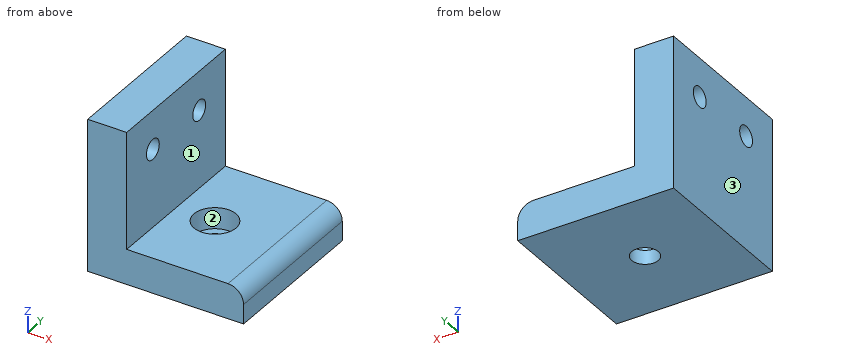
```python
from build123d import *

# Parameters (mm, degrees)
SKETCH_W        = 20
SKETCH_H        = 20
PAD_DEPTH       = 4.5
SKETCH001_R     = 1.7
POCKET_DEPTH    = 5
SKETCH002_R     = 2.7
POCKET001_DEPTH = 2.7
SKETCH003_W     = 5
SKETCH003_H     = 20
PAD001_DEPTH    = 15
SKETCH004_R     = 1.3
POCKET002_DEPTH = 5
FILLET_R        = 2


with BuildPart() as part:
    # Sketch → Pad (new body)
    with BuildSketch(Plane.XY):
        Rectangle(SKETCH_W, SKETCH_H)
    extrude(amount=PAD_DEPTH)

    # Sketch001 (on Face6 of Pad) → Pocket (cut)
    with BuildSketch(Plane.XY.offset(4.5)):
        Circle(SKETCH001_R)
    extrude(amount=-POCKET_DEPTH, mode=Mode.SUBTRACT)

    # Sketch002 (on Face5 of Pocket) → Pocket001 (cut)
    with BuildSketch(Plane.XY.offset(4.5)):
        Circle(SKETCH002_R)
    extrude(amount=-POCKET001_DEPTH, mode=Mode.SUBTRACT)

    # Sketch003 (on Face5 of Pocket001) → Pad001 (join)
    with BuildSketch(Plane.XY.offset(4.5)):
        with Locations((-7.5, 0)):
            Rectangle(SKETCH003_W, SKETCH003_H)
    extrude(amount=PAD001_DEPTH)

    # Sketch004 (on Face10 of Pad001) → Pocket002 (cut)
    with BuildSketch(Plane.YZ.offset(-5)):
        with Locations((-4.7, 14.5)):
            Circle(SKETCH004_R)
        with Locations((4.7, 14.5)):
            Circle(SKETCH004_R)
    extrude(amount=-POCKET002_DEPTH, mode=Mode.SUBTRACT)

    # Fillet
    fillet_edges = [part.edges().sort_by_distance(p)[0] for p in [
        (10, 0, 4.5),
    ]]
    fillet(fillet_edges, radius=FILLET_R)


solid = part.part
```
Here's how the part is built. I have some questions about the finished solid (model axes, mm). Face numbers are marked on the shaded views. A direction names the side the tool comes from. Coordinates: 2 decimals unless noted, no trailing zeros. Order: outer loops, then holes, each group sorted by start corner. A loop starts at its lowest first (then second) coordinate and runs counter-clockwise, first axis right, second up.
1) Will these pins go through, and if not, where does the flat tip stop? pin 1 (8 mm diameter, centred on x = 3, y = -6.5, fed in from +Z); pin 2 (7.5 mm diameter, centred on y = 2.5, z = 13, fed in from +X).
2) I need wall thicknesses on line 1 (Y direction, x = 0, z = 1.15); line 2 (Y direction, x = 0, z = 3); line 3 (Z direction, x = -8, y = 4.7). Which ranges of each line are inside material? Lowest first, please.
3) Imagine slicing it at C-C on z = 14.5. List the corners of the cut face in (x, y) for me.
4) Imagine slicing it at B-B on x = 0. List the corners of the cut face in (y, z) for me, and give its area (3 significant figures).
5) Which directions (+Z, -Z, +X, -X, +Y, -Y) give clear straight access to the entire face, cutting with the end or side of a thin tool? Please do the marked faces 1, 2 and 3.
6) Imagine slicing it at D-D on x = -6.75. List the corners of the cut face in (y, z) for me, and give its area (3 significant figures).
7) Imagine slicing it at A-A on y = -4.7. List the corners of the cut face in (x, z) for me, and give its area (3 significant figures).
Response values:
1. pin 1: stops at z = 4.5
1. pin 2: stops at x = -5
2. line 1: y = -10 to -1.7, 1.7 to 10
2. line 2: y = -10 to -2.7, 2.7 to 10
2. line 3: z = 0 to 13.2, 15.8 to 19.5
3. outline: (-10, -10) - (-5, -10) - (-5, -6) - (-10, -6) - close; (-10, -3.4) - (-5, -3.4) - (-5, 3.4) - (-10, 3.4) - close; (-10, 6) - (-5, 6) - (-5, 10) - (-10, 10) - close
4. outline: (-10, 0) - (-1.7, 0) - (-1.7, 1.8) - (-2.7, 1.8) - (-2.7, 4.5) - (-10, 4.5) - close; (1.7, 0) - (10, 0) - (10, 4.5) - (2.7, 4.5) - (2.7, 1.8) - (1.7, 1.8) - close
4. area: 69.3 mm2
5. face 1: +Z, +X, +Y, -Y
5. face 2: +Z
5. face 3: +Z, -Z, -X, +Y, -Y
6. outline: (-10, 0) - (10, 0) - (10, 19.5) - (-10, 19.5) - close; hole circle Ø2.6 at (-4.7, 14.5); hole circle Ø2.6 at (4.7, 14.5)
6. area: 379 mm2
7. outline: (-10, 0) - (10, 0) - (10, 2.5) arc R2 ccw to (8, 4.5) - (-5, 4.5) - (-5, 13.2) - (-10, 13.2) - close; (-10, 15.8) - (-5, 15.8) - (-5, 19.5) - (-10, 19.5) - close
7. area: 151 mm2
